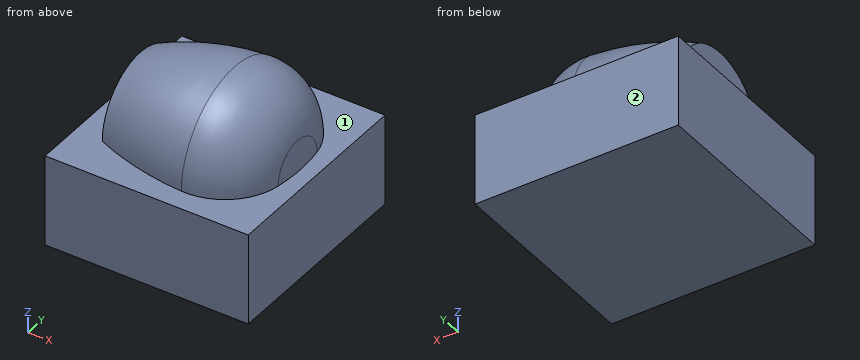
from build123d import *

# Parameters (mm, degrees)
F2_W     = 113.065446
F2_H     = 114.160227
F3_DEPTH = 50.8


with BuildPart() as f1:
    # F0 (on Top) → F1 (revolve)
    with BuildSketch(Plane.XY):
        with BuildLine():
            Line((0, -31.75), (88.9, -31.75))
            ThreePointArc((88.9, -31.75), (88.56236, -23.579488), (87.551741, -15.464692))
            ThreePointArc((87.551741, -15.464692), (75.365793, 5.308771), (52.427336, 12.647797))
            ThreePointArc((52.427336, 12.647797), (25.639597, 8.703524), (0, 0))
            Line((0, 0), (0, -31.75))
        make_face()
    revolve(axis=Axis((44.45, -31.75, 0), (-1, 0, 0)))

    # F2 (on Top) → F3 (join)
    with BuildSketch(Plane.XY):
        with Locations((40.961946, -30.810474)):
            Rectangle(F2_W, F2_H)
    extrude(amount=-F3_DEPTH)


solid = f1.part
Geometry check sheet. Reference: the model listing, model coordinates, mm. Face numbers are marked on the shaded views. A direction names the side the tool comes from. Give positions to 0.01 mm unless a question says otherwise; leave off trailing zeros. Order: outer loops, then holes, each group sorted by start corner. A loop starts at its lowest first (then second) coordinate and runs counter-clockwise, first axis right, second up.
1) Material ranges on probe 1 along Z at (x, y) = (-6, 13); probe 2 along X at (y, z) = (-42.5, 12); probe 3 along Z at (x, y) = (62.5, -72), recorded low to high.
Results are:
probe 1: z = -50.8 to 0
probe 2: x = 0 to 87.58
probe 3: z = -50.8 to 16.33
2) Cross-section at A-A (y = -78). Record the boundary of the cut face in (x, z), then the cut area to 3 significant figures.
Results are:
outline: (-15.57, -50.8) - (97.49, -50.8) - (97.49, 0) - (-15.57, 0) - close
area: 5,740 mm2
3) Gauge pin test, flat ends, axial feed: pin 1 (4 mm diameter, centred on x = 44.5, y = -38, fed in from +Z); pin 2 (12 mm diameter, centred on x = 32, y = -67.5, fed in from +Z); pin 3 (4 mm diameter, centred on y = -15, z = 21.5, fed in from +X). Record the tip position at first contact, or that the pin passes through.
Results are:
pin 1: stops at z = 43.63
pin 2: stops at z = 29.64
pin 3: stops at x = 84.73
4) Tool access check on the marked faces 1 and 2. Record the directions out of +Z, -Z, +X, -X, +Y, -Y that give a thin tool (end or side, any length) a straight path to the whole face; none if there is none.
Results are:
face 1: +Z
face 2: +Z, -Z, +X, -X, +Y
